For this review, take the finished solid that the model builds, in its own axes (mm). Face numbers are marked on the shaded views. A direction names the side the tool comes from. Coordinates: 2 decimals unless noted, no trailing zeros. Loops run counter-clockwise (first coordinate to the right, second up) from the corner with the lowest first, then second, coordinate; pieces in that order, holes last. Notation, with made-up numbers: (76.25, -8) - (98.25, -8) arc R25 cw to (98.25, 24) - close; hole circle Ø11 at (39, -12). An arc over 180 degrees is marked (long way). One line per item, written item: value. Start each with the question number.
1. For the marked faces 1, 2 and 3, list the 3-axis set-ups (+Z, -Z, +X, -X, +Y, -Y) from which the entire face can be reached by the end or side of a thin tool; tool diameter is ignored.
2. To check wall thickness, follow line 1 (Y direction, x = 0, z = 135.5); line 2 (X direction, y = 12.5, z = 28.5); line 3 (Y direction, x = 0, z = 7). State the ranges of each line that lie inside material, in increasing order. Write a range as from..to.
3. Take a section at B-B, the plane x = 0. Count the separate pieces of the cut face and the enclosed holes in it, and give its area (3 significant figures).
4. Insertion check: pin 1 (10 mm diameter, centred on y = 1.5, z = 24.5, fed in from -X); pin 2 (21.5 mm diameter, centred on x = -4, z = 117.5, fed in from +Y). Each pin has a flat end and moves straight along its axis. Give the tip position at first contact, or say it passes through.
5. Take a section at A-A, the plane z = 58.5. State the section outline as (x, y) points.
6. Take a section at D-D, the plane z = 72.5. State the section outline as (x, y) points, and give its area (3 significant figures).
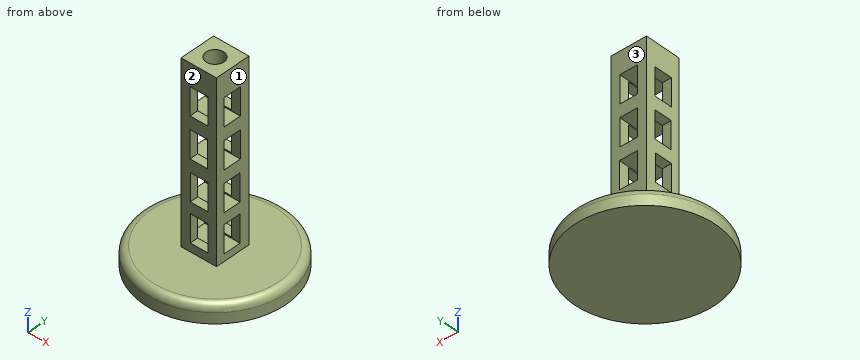
```python
from build123d import *

# Parameters (mm, degrees)
F0_R     = 50.8
F1_DEPTH = 12.7
F2_W     = 25.4
F2_H     = 25.4
F3_DEPTH = 127
F4_W     = 12.7
F4_H     = 19.730706
F5_DEPTH = 25.4
F6_W     = 12.7
F6_H     = 19.730706
F7_DEPTH = 25.4
F8_R     = 6.35
F9_DEPTH = 12.7
F10_R    = 5.08


with BuildPart() as f1:
    # F0 (on Top) → F1 (new body)
    with BuildSketch(Plane.XY):
        Circle(F0_R)
    extrude(amount=F1_DEPTH)

    # F2 (on face) → F3 (join)
    with BuildSketch(Plane.XY.offset(12.7)):
        Rectangle(F2_W, F2_H)
    extrude(amount=F3_DEPTH)

    # F4 (on face) → F5 (cut)
    with BuildSketch(Plane.XZ.offset(12.7)):
        with Locations((0.098038, 113.95823)):
            Rectangle(F4_W, F4_H)
        with Locations((0.036561, 85.036777)):
            Rectangle(F4_W, F4_H)
        with Locations((0.27161, 56.256354)):
            Rectangle(F4_W, F4_H)
        with Locations((0.271611, 28.572757)):
            Rectangle(F4_W, F4_H)
    extrude(amount=-F5_DEPTH, mode=Mode.SUBTRACT)

    # F6 (on face) → F7 (cut)
    with BuildSketch(Plane(origin=(-12.7, 0, 0), x_dir=(0, -1, 0), z_dir=(-1, 0, 0))):
        with Locations((0.396478, 113.09307)):
            Rectangle(F6_W, F6_H)
        with Locations((0.335001, 84.171617)):
            Rectangle(F6_W, F6_H)
        with Locations((0.57005, 55.391194)):
            Rectangle(F6_W, F6_H)
        with Locations((0.570051, 27.707597)):
            Rectangle(F6_W, F6_H)
    extrude(amount=-F7_DEPTH, mode=Mode.SUBTRACT)

    # F8 (on face) → F9 (cut)
    with BuildSketch(Plane.XY.offset(139.7)):
        Circle(F8_R)
    extrude(amount=-F9_DEPTH, mode=Mode.SUBTRACT)

    # F10
    f10_edges = [f1.edges().sort_by_distance(p)[0] for p in [
        (-50.8, 0, 12.7),
    ]]
    fillet(f10_edges, radius=F10_R)


solid = f1.part
```
Solutions:
1. face 1: +Z, +X, +Y, -Y
1. face 2: +Z, +X, -X, -Y
1. face 3: +Z, +X, -X, +Y
2. line 1: -12.7..-6.35, 6.35..12.7
2. line 2: -12.7..-6.08, 6.62..12.7
2. line 3: -50.8..50.8
3. separate pieces: 5
3. enclosed holes: 0
3. area: 2,300 mm2
4. pin 1: x = -12.7
4. pin 2: y = 12.7
5. outline: (-12.7, -12.7) - (-6.08, -12.7) - (-6.08, -6.92) - (-12.7, -6.92) - close; (-12.7, 5.78) - (-6.08, 5.78) - (-6.08, 12.7) - (-12.7, 12.7) - close; (6.62, -12.7) - (12.7, -12.7) - (12.7, -6.92) - (6.62, -6.92) - close; (6.62, 5.78) - (12.7, 5.78) - (12.7, 12.7) - (6.62, 12.7) - close
6. outline: (-12.7, -12.7) - (12.7, -12.7) - (12.7, 12.7) - (-12.7, 12.7) - close
6. area: 645 mm2
